Could you check a few things on this model? Use its own coordinates, in mm. Give positions to 0.01 mm unless a question says otherwise; leave off trailing zeros. Loops run counter-clockwise (first coordinate to the right, second up) from the corner with the lowest first, then second, coordinate; pieces in that order, holes last. Notation, with made-up numbers: (-9.5, -12.5) - (31.5, -12.5) arc R23 cw to (31.5, 25.5) - close; hole circle Ø11 at (-7.75, 3.25). An arc over 180 degrees is marked (long way). Write each question's results on one line, items separated by ' | '. Start each with the question number.
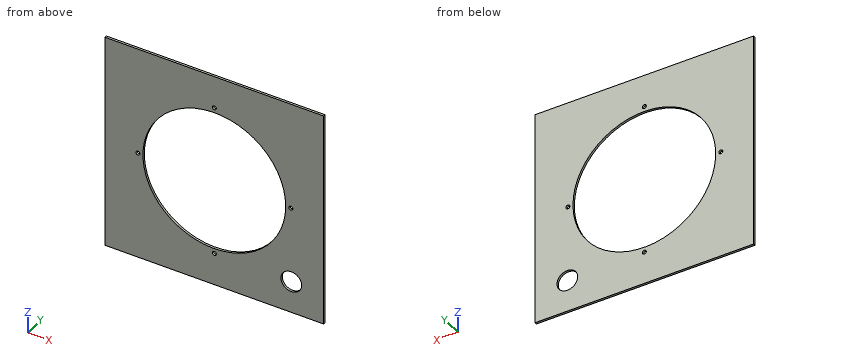
```python
from build123d import *

# Parameters (mm, degrees)
SKETCH1_W           = 300
SKETCH1_H           = 300
BOSS_EXTRUDE1_DEPTH = 3
CUT_EXTRUDE1_REACH  = 5
SKETCH2_R           = 98
SKETCH2_R_2         = 14.255
SKETCH4_R           = 2.75
CUT_EXTRUDE3_DEPTH  = 4


with BuildPart() as part:
    # Sketch1 → Boss-Extrude1 (new body)
    with BuildSketch(Plane(origin=(0, 0, 0), x_dir=(1, 0, 0), z_dir=(0, 1, 0))):
        with Locations((150, -150)):
            Rectangle(SKETCH1_W, SKETCH1_H)
    extrude(amount=BOSS_EXTRUDE1_DEPTH)

    # Sketch2 → Cut-Extrude1 (cut, up to next)
    with BuildSketch(Plane(origin=(0, 3, 0), x_dir=(1, 0, 0), z_dir=(0, 1, 0)), mode=Mode.PRIVATE) as cut_extrude1_sk1:
        with Locations((150, -150)):
            Circle(SKETCH2_R)
    cut_extrude1_tool1 = extrude(cut_extrude1_sk1.sketch, amount=-CUT_EXTRUDE1_REACH, mode=Mode.PRIVATE) & part.part
    add(cut_extrude1_tool1.solids().sort_by_distance((150, 3, 150))[0], mode=Mode.SUBTRACT)
    # Sketch2 → Cut-Extrude1 (cut, up to next)
    with BuildSketch(Plane(origin=(0, 3, 0), x_dir=(1, 0, 0), z_dir=(0, 1, 0)), mode=Mode.PRIVATE) as cut_extrude1_sk2:
        with Locations((255.712463787, -44.287536213)):
            Circle(SKETCH2_R_2)
    cut_extrude1_tool2 = extrude(cut_extrude1_sk2.sketch, amount=-CUT_EXTRUDE1_REACH, mode=Mode.PRIVATE) & part.part
    add(cut_extrude1_tool2.solids().sort_by_distance((255.712464, 3, 44.287536))[0], mode=Mode.SUBTRACT)

    # Sketch4 → Cut-Extrude3 (cut, through all)
    with BuildSketch(Plane(origin=(0, 3, 0), x_dir=(1, 0, 0), z_dir=(0, 1, 0))):
        with Locations((45, -150)):
            Circle(SKETCH4_R)
        with Locations((255, -150)):
            Circle(SKETCH4_R)
        with Locations((150, -255)):
            Circle(SKETCH4_R)
        with Locations((150, -45)):
            Circle(SKETCH4_R)
    extrude(amount=-CUT_EXTRUDE3_DEPTH, mode=Mode.SUBTRACT)


solid = part.part
```
Q1. I need wall thicknesses on L1, parallel to Z at x = 255, y = 1.65; L2, parallel to Z at x = 150, y = 1.25. Which ranges of each line are inside material? Lowest first, please. Write a range as from..to.
Q2. I want a section at B-B, the plane x = 64. List the corners of the cut face in (y, z) for me.
Q3. I want a section at A-A, the plane z = 81. List the corners of the cut face in (x, y) for me.
Q4. I want a section at C-C, the plane y = 0.5. List the corners of the cut face in (x, z) for me (3 decimals), then the cut area to 3 significant figures.
Q5. I'm going to push flat-ended pins straight in: pin 1 Ø4.5 at (x, z) = (255, 150) entering from -Y; pin 2 Ø1 at (y, z) = (1.5, 94) entering from -X. Where does each tip first touch, or does it pass through?
Conclusion:
1) L1: 0..30.05, 58.52..147.25, 152.75..300 | L2: 0..42.25, 47.75..52, 248..252.25, 257.75..300
2) outline: (0, 0) - (3, 0) - (3, 103.01) - (0, 103.01) - close; (0, 196.99) - (3, 196.99) - (3, 300) - (0, 300) - close
3) outline: (0, 0) - (80.41, 0) - (80.41, 3) - (0, 3) - close; (219.59, 0) - (300, 0) - (300, 3) - (219.59, 3) - close
4) outline: (0, 0) - (300, 0) - (300, 300) - (0, 300) - close; hole circle Ø5.5 at (45, 150); hole circle Ø196 at (150, 150); hole circle Ø5.5 at (150, 45); hole circle Ø5.5 at (150, 255); hole circle Ø28.51 at (255.712, 44.288); hole circle Ø5.5 at (255, 150) | area: 59,100 mm^2
5) pin 1: through | pin 2: x = 0
